Geometry check sheet. Reference: drawing and pictorial views, mm from the part's lowest x, y, z. A direction names the side the tool comes from. Give positions to 0.01 mm unless a question says otherwise; leave off trailing zeros. Write each loop counter-clockwise with the first axis right and the second up, starting at its lowest first coordinate (ties: lowest second). Pieces come first, ordered by that corner, then holes.
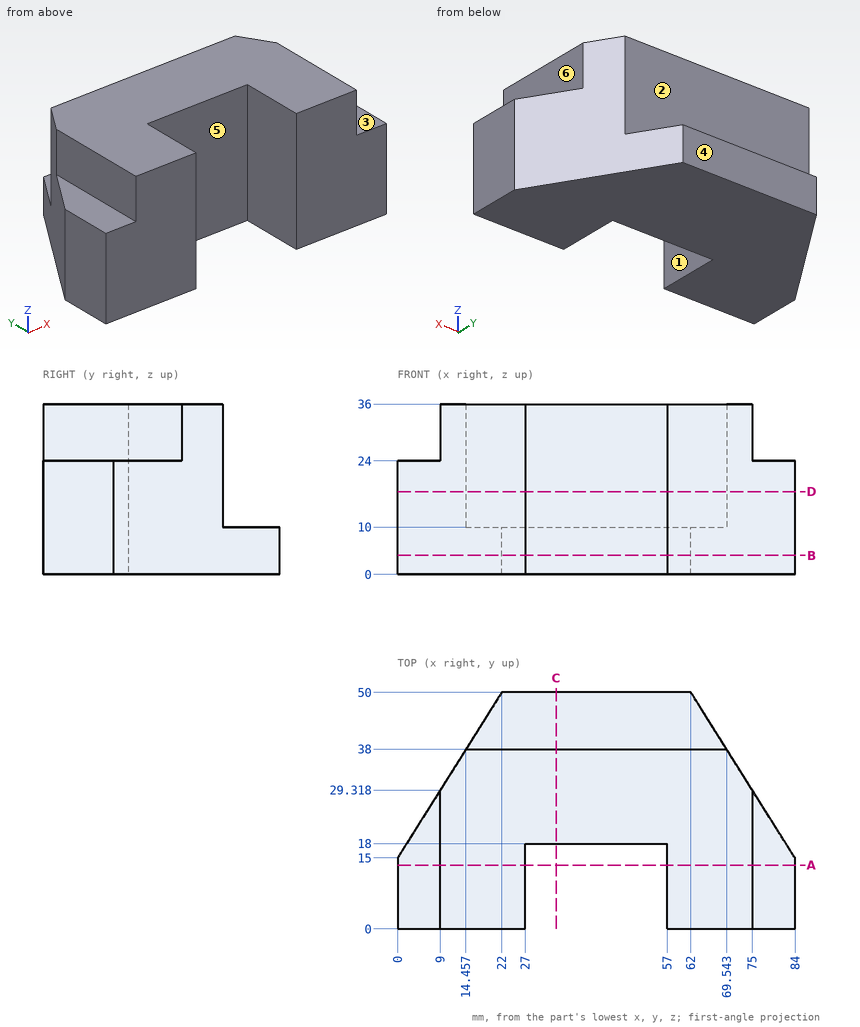
Item 1: Sectioned sample at B-B on z = 4. Record the cut outline in (x, y), then the cut area to 3 significant figures.
Answer key:
outline: (0, 0) - (27, 0) - (27, 18) - (57, 18) - (57, 0) - (84, 0) - (84, 15) - (62, 50) - (22, 50) - (0, 15) - close
area: 2,890 mm2
Item 2: Scan lines: line 1 along X through (y, z) = (2, 19); line 2 along X through (y, z) = (9, 31.5); line 3 along Y through (x, z) = (44, 21). Record each from-to range of solid material in increasing order.
Answer key:
line 1: x = 0 to 27, 57 to 84
line 2: x = 9 to 27, 57 to 75
line 3: y = 18 to 38
Item 3: Sectioned sample at D-D on z = 17.5. Record the cut outline in (x, y), then the cut area to 3 significant figures.
Answer key:
outline: (0, 0) - (27, 0) - (27, 18) - (57, 18) - (57, 0) - (84, 0) - (84, 15) - (69.54, 38) - (14.46, 38) - (0, 15) - close
area: 2,320 mm2
Item 4: Depth check by flat-ended pin: pin 1 (5 mm diameter, centred on x = 32, z = 22, fed in from -Y); pin 2 (13 mm diameter, centred on x = 41.5, y = 42, fed in from +Z); pin 3 (1.5 mm diameter, centred on y = 32, z = 11, fed in from -X); pin 4 (4 mm diameter, centred on x = 45.5, z = 28, fed in from +Y). Enter the tip coordinate at first touch or a pass-through.
Answer key:
pin 1: stops at y = 18
pin 2: stops at z = 36
pin 3: stops at x = 10.21
pin 4: stops at y = 38
Item 5: Sectioned sample at C-C on x = 33.5. Record the cut outline in (y, z), then the cut area to 3 significant figures.
Answer key:
outline: (18, 0) - (50, 0) - (50, 10) - (38, 10) - (38, 36) - (18, 36) - close
area: 840 mm2
Item 6: Release check for a two-part mould opening along X. For the marked faces 4, 5 and 6 record: released by +X, released by -X, zero draft, split by the parting line, or undercut.
Answer key:
face 4: zero draft
face 5: undercut
face 6: released by +X
Item 7: Set-up check for the marked faces 1, 2 and 3: record each of +Z, -Z, +X, -X, +Y, -Y from which the full face is reachable in a straight line by a thin tool's end or side.
Answer key:
face 1: +Z, -Z, -Y
face 2: +Z, +X, -X, +Y
face 3: +Z, +X, +Y, -Y
Item 8: Sectioned sample at A-A on y = 13.5. Record the cut outline in (x, z), then the cut area to 3 significant figures.
Answer key:
outline: (0, 0) - (27, 0) - (27, 36) - (9, 36) - (9, 24) - (0, 24) - close; (57, 0) - (84, 0) - (84, 24) - (75, 24) - (75, 36) - (57, 36) - close
area: 1,730 mm2
